```python
from build123d import *

# Parameters (mm, degrees)
SKETCH_1_R               = 5.06
SKETCH_1_R_2             = 1.7
EXTRUDE_2_DEPTH          = 30
CUT_EXTRUDE_1_DEPTH      = 63.561467357
CUT_EXTRUDE_1_DEPTH_BACK = 63.561467357
SKETCH_3_R               = 2.1
CUT_EXTRUDE_2_DEPTH      = 62.283268979
CUT_EXTRUDE_2_DEPTH_BACK = 3.5
SKETCH_6_R               = 10.85
SKETCH_7_R               = 10.85
CUT_EXTRUDE_3_DEPTH      = 3.5
SKETCH_8_R               = 2
CUT_EXTRUDE_4_DEPTH      = 10


with BuildPart() as part:
    # Эскиз1 → Бобышка-Вытянуть2 (new body)
    with BuildSketch(Plane(origin=(0, 0, 0), x_dir=(0, 0, -1), z_dir=(1, 0, 0))):
        Polygon((15.028471622, 20.43775572), (15.028471622, -3.56224428), (49.375471622, -3.56224428), (49.375471622, -9.56224428), (-49.318528378, -9.56224428), (-49.318528378, -3.56224428), (-14.971528378, -3.56224428), (-14.971528378, 20.43775572), align=None)
        with Locations((-0.246661602, 8.38775572)):
            Circle(SKETCH_1_R, mode=Mode.SUBTRACT)
        with Locations((7.363604846, 8.38775572)):
            Circle(SKETCH_1_R_2, mode=Mode.SUBTRACT)
        with Locations((-7.306661602, 8.38775572)):
            Circle(SKETCH_1_R_2, mode=Mode.SUBTRACT)
    extrude(amount=EXTRUDE_2_DEPTH)

    # Эскиз3 → Вырез-Вытянуть1 (cut, two sides: drawn at the far end of the back side and taken through both)
    with BuildSketch(Plane(origin=(0, -3.56224428, 0), x_dir=(1, 0, 0), z_dir=(0, 1, 0)).offset(-CUT_EXTRUDE_1_DEPTH_BACK)):
        with Locations(Location((6, -20.318528378, 0), (0, 0, 270))):
            Circle(SKETCH_3_R)
        with Locations(Location((24, -20.318528378, 0), (0, 0, 270))):
            Circle(SKETCH_3_R)
        with Locations(Location((24, -44.318528378, 0), (0, 0, 270))):
            Circle(SKETCH_3_R)
        with Locations(Location((6, -44.318528378, 0), (0, 0, 270))):
            Circle(SKETCH_3_R)
        with Locations(Location((6, 44.375471622, 0), (0, 0, 90))):
            Circle(SKETCH_3_R)
        with Locations(Location((24, 44.375471622, 0), (0, 0, 90))):
            Circle(SKETCH_3_R)
        with Locations(Location((24, 20.375471622, 0), (0, 0, 90))):
            Circle(SKETCH_3_R)
        with Locations(Location((6, 20.375471622, 0), (0, 0, 90))):
            Circle(SKETCH_3_R)
    extrude(amount=CUT_EXTRUDE_1_DEPTH + CUT_EXTRUDE_1_DEPTH_BACK, mode=Mode.SUBTRACT)

    # Эскиз6 → Вырез-Вытянуть2 (cut, two sides: drawn at the far end of the back side and taken through both)
    with BuildSketch(Plane(origin=(30, 0, 0), x_dir=(0, 0, -1), z_dir=(1, 0, 0)).offset(-CUT_EXTRUDE_2_DEPTH_BACK)):
        with Locations(Location((-0.067919336, 8.365106346, 0), (0, 0, 180))):
            Circle(SKETCH_6_R)
    extrude(amount=CUT_EXTRUDE_2_DEPTH + CUT_EXTRUDE_2_DEPTH_BACK, mode=Mode.SUBTRACT)

    # Эскиз7 → Вырез-Вытянуть3 (cut)
    with BuildSketch(Plane.ZY):
        with Locations((0.246661602, 8.38775572)):
            Circle(SKETCH_7_R)
    extrude(amount=-CUT_EXTRUDE_3_DEPTH, mode=Mode.SUBTRACT)

    # Эскиз8 → Вырез-Вытянуть4 (cut)
    with BuildSketch(Plane(origin=(0, 20.43775572, 0), x_dir=(1, 0, 0), z_dir=(0, 1, 0))):
        with Locations(Location((6.529067928, 11.609424623, 0), (0, 0, 270))):
            Circle(SKETCH_8_R)
        with Locations(Location((23.470932072, 11.609424623, 0), (0, 0, 90))):
            Circle(SKETCH_8_R)
        with Locations(Location((23.492925715, -11.564853382, 0), (0, 0, 270))):
            Circle(SKETCH_8_R)
        with Locations(Location((6.55109209, -11.597010844, 0), (0, 0, 90))):
            Circle(SKETCH_8_R)
    extrude(amount=-CUT_EXTRUDE_4_DEPTH, mode=Mode.SUBTRACT)


solid = part.part
```
Geometry: final body of the model. Coordinates: model frame, mm. A direction names the side the tool comes from. Round coordinates to 2 decimals unless told otherwise and drop trailing zeros. Order: outer loops, then holes, each group sorted by start corner. A loop starts at its lowest first (then second) coordinate and runs counter-clockwise, first axis right, second up. Notation, with made-up numbers: (27.5, 70.25) -> (64.5, 70.25) arc R28 ccw to (64.5, 98.25) -> close; hole circle Ø11 at (13.25, 68.25). An arc over 180 degrees is marked (long way). Use CSV: the item, a comma, the result in double quotes. Start each with the question number.
1) Section A-A (y = -4.5). State how many separate pieces and enclosed holes the cut face has, and give its area (3 significant figures).
2) Section B-B (z = 3.5). Return the cut outline in (x, y).
3) Section D-D (z = -19.5). Return the cut outline in (x, y), and give its area (3 significant figures).
4) First-contact query: pin 1 Ø6 at (y, z) = (-2, 27.5) entering from +X; pin 2 Ø3 at (x, z) = (23.5, -12) entering from +Y; pin 3 Ø1 at (x, z) = (10, 32.5) entering from +Y; pin 4 Ø2.5 at (y, z) = (8.39, -7.36) entering from +X. Flat tips, straight axial feed; report the tip coordinate or a pass-through.
5) Draft query along X for faces 1 (the face through (25.42, -6.6, 42.77)), 2 (the face through (3.5, 6, 5)), 3 (the face through (1.726, 11.647, 10.596)), 4 (the face through (30, -4, -1)). Return one class per face: +X half, -X half, draft (parallel to the pull), parting line (faces both ways), or undercut.
6) Material intervals for line 1 along Z through (x, y) = (14.75, 8.5); line 2 along Z through (x, y) = (23, 11.5); line 3 along Z through (x, y) = (19.5, 1.5), sorted ascending. Write a range as from..to.
7) Set-up query: faces 5 (the face through (15, 20.438, 0)), 6 (the face through (24, 10.438, 12)), 7 (the face through (28.23, 5.11, 10.42)), 8 (the face through (14.839, 7.737, -8.934)), 9 (the face through (15, 8, 14.972)). Return all of +Z, -Z, +X, -X, +Y, -Y with unobstructed straight access to the full face (end or side cutting, diameter ignored); none if empty.
8) Section C-C (y = 15). Return the cut outline in (x, z).
Returned:
1,separate pieces,"1"
1,enclosed holes,"8"
1,area,"2,850 mm²"
2,outline,"(0, -9.56) -> (30, -9.56) -> (30, -1.93) -> (26.5, -1.93) -> (26.5, 4.51) -> (3.5, 4.51) -> (3.5, -1.96) -> (0, -1.96) -> close; (0, 18.74) -> (3.5, 18.74) -> (3.5, 12.26) -> (26.5, 12.26) -> (26.5, 18.66) -> (30, 18.66) -> (30, 20.44) -> (0, 20.44) -> close"
3,outline,"(0, -9.56) -> (4.09, -9.56) -> (4.09, -3.56) -> (0, -3.56) -> close; (7.91, -9.56) -> (22.09, -9.56) -> (22.09, -3.56) -> (7.91, -3.56) -> close; (25.91, -9.56) -> (30, -9.56) -> (30, -3.56) -> (25.91, -3.56) -> close"
3,area,"134 mm²"
4,pin 1,"stops at x = 30"
4,pin 2,"stops at y = 10.44"
4,pin 3,"stops at y = -3.56"
4,pin 4,"passes through"
5,face 1,"undercut"
5,face 2,"-X half"
5,face 3,"draft"
5,face 4,"+X half"
6,line 1,"z = -15.03..-9.06, -5.67..-4.81, 5.31..5.61, 9..14.97"
6,line 2,"z = -15.03..-13.55, -9.67..-3.74, 4.24..9.63, 13.5..14.97"
6,line 3,"z = -15.03..14.97"
7,face 5,"+Z, -Z, +X, -X, +Y"
7,face 6,"+Y"
7,face 7,"+X"
7,face 8,"+X, -X"
7,face 9,"+Z, +X, -X, +Y"
8,outline,"(0, -15.03) -> (30, -15.03) -> (30, -8.52) -> (26.5, -8.52) -> (26.5, 8.65) -> (30, 8.65) -> (30, 14.97) -> (0, 14.97) -> (0, 8.85) -> (3.5, 8.85) -> (3.5, -8.36) -> (0, -8.36) -> close; hole circle Ø4 at (6.53, -11.61); hole circle Ø4 at (6.55, 11.6); hole circle Ø4 at (23.47, -11.61); hole circle Ø4 at (23.49, 11.56)"
